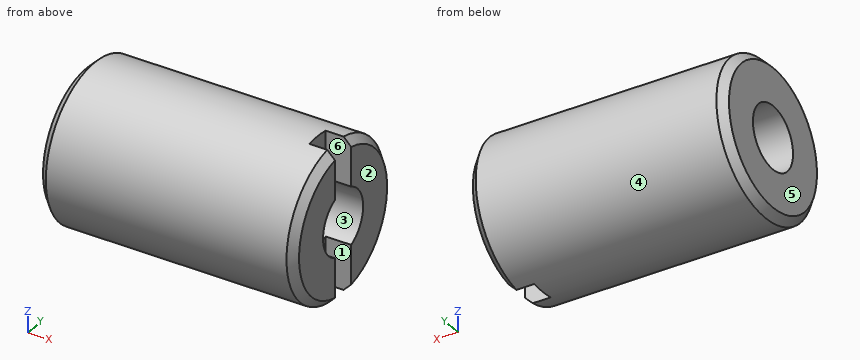
Autodesk Inventor part; units mm, degrees
ref_plane "YZ Plane" through (0, 0, 0) normal (1, 0, 0) x (0, 1, 0)
ref_plane "XZ Plane" through (0, 0, 0) normal (0, 1, 0) x (-1, 0, 0)
ref_plane "XY Plane" through (0, 0, 0) normal (0, 0, 1) x (1, 0, 0)
sketch "スケッチ1" plane through (0, 0, 0) normal (0, 1, 0) x (-1, 0, 0)
  line L0 (0, 0) -> (10, 0)
  line L1 (10, 0) -> (10, -3)
  line L2 (10, -3) -> (0, -3)
  line L3 (0, -3) -> (0, 0)
  dimension "d0" = 10
  dimension "d1" = 3
revolve "回転1" add sketch "スケッチ1" angle 360 about axis through (0, 0, 0) along (-1, 0, 0)
sketch "スケッチ2" plane through (0, 0, 0) normal (1, 0, 0) x (0, 0, -1)
  point P0 (0, 0)
  point P1 (0, 0)
hole "穴1" at (0, 0, 0) direction (-1, 0, 0) diameter 2.459 end through all
sketch "スケッチ3" plane through (0, 0, 0) normal (1, 0, 0) x (0, 0, -1)
  circle A0 centre (0, 0) radius 3
  line L0 (3, 0) -> (-3, 0)
  line L1 (3, -0.5) -> (-3, -0.5)
  line L2 (3, 0.5) -> (-3, 0.5)
  line L3 (3, 0.5) -> (3, -0.5)
  line L4 (-3, 0.5) -> (-3, -0.5)
  point P0 (-2.958, -0.5)
  point P1 (2.958, -0.5)
  point P2 (2.958, 0.5)
  point P3 (-2.958, 0.5)
  dimension "d10" = 0.5
extrude "押し出し1" cut sketch "スケッチ3" against normal blind 1 contours L0 A0 L2 | A0 L1 L0
chamfer "面取り1" distance 0.3 angle 45 3 edges at (-10, 0, 3) (0, 3, 0) (0, -3, 0)
properties part number "ARU-3010S" material "ステンレス鋼 440C"
Work out the finished part from the listing and answer in its coordinate system (mm). Face numbers are marked on the shaded views. A direction names the side the tool comes from. Round coordinates to 2 decimals unless told otherwise and drop trailing zeros. Write each loop counter-clockwise with the first axis right and the second up, starting at its lowest first coordinate (ties: lowest second). Pieces come first, ordered by that corner, then holes. Notation, with made-up numbers: (-32, 21) - (-9, 21) arc R30 ccw to (-9, 56) - close; hole circle Ø5 at (42, 39). An arc over 180 degrees is marked (long way). Return JSON: item names as keys, results as strings. Group by question number.
Q1. The mould has two halves that part along Y. Classify the marked faces 1, 2, 3 and 4: released by +Y, released by -Y, zero draft, split by the parting line, or undercut.
Q2. The part is cut by section A-A on z = 0. Write down the section's boundary in (x, y).
Q3. The part is cut by section C-C on x = -5. Write down the section's boundary in (y, z), then the cut area to 3 significant figures.
Q4. Find the intervals of material crossed by L1, parallel to Y at x = -9.5, z = 0.5; L2, parallel to Z at x = -8, y = 0, in increasing order.
Q5. For the marked faces 5 and 6, determine the directions among +Z, -Z, +X, -X, +Y, -Y from which every point of the face is accessible in a straight line to the end or side of a thin tool.
Q6. Each of these flat-tipped pins is pushed along its axis until it touches: pin 1 Ø1.5 at (x, z) = (-3, 2) entering from +Y; pin 2 Ø3 at (y, z) = (0, 0) entering from -X; pin 3 Ø1 at (x, z) = (-8, 1.5) entering from +Y; pin 4 Ø1.1 at (x, z) = (-0.5, -2.5) entering from -Y. Where does it stop, or does it pass through?
Q7. The part is cut by section B-B on y = 0. Write down the section's boundary in (x, z), then the cut area to 3 significant figures.
Solved:
{
 "1": {"face 1": "undercut", "face 2": "zero draft", "face 3": "undercut", "face 4": "split by the parting line"},
 "2": {"outline": "(-10, -2.7) - (-9.7, -3) - (-0.3, -3) - (0, -2.7) - (0, -1.23) - (-10, -1.23) - close; (-10, 1.23) - (0, 1.23) - (0, 2.7) - (-0.3, 3) - (-9.7, 3) - (-10, 2.7) - close"},
 "3": {"outline": "circle Ø6 at (0, 0); hole circle Ø2.46 at (0, 0)", "area": "23.5 mm²"},
 "4": {"L1": "-2.96 to -1.12, 1.12 to 2.96", "L2": "-3 to -1.23, 1.23 to 3"},
 "5": {"face 5": "+Z, -Z, -X, +Y, -Y", "face 6": "+Z, -Z, +X"},
 "6": {"pin 1": "y = 2.73", "pin 2": "x = -10", "pin 3": "y = 2.83", "pin 4": "y = -2.28"},
 "7": {"outline": "(-10, -2.7) - (-9.7, -3) - (-1, -3) - (-1, -1.23) - (-10, -1.23) - close; (-10, 1.23) - (-1, 1.23) - (-1, 3) - (-9.7, 3) - (-10, 2.7) - close", "area": "31.8 mm²"}
}
